For this review, take the finished solid that the model builds, in its own axes (mm). Face numbers are marked on the shaded views. A direction names the side the tool comes from. Give positions to 0.01 mm unless a question says otherwise; leave off trailing zeros. Loops run counter-clockwise (first coordinate to the right, second up) from the corner with the lowest first, then second, coordinate; pieces in that order, holes last.
```python
from build123d import *

# Parameters (mm, degrees)
CROQUIS1_R              = 4
SALIENTE_EXTRUIR1_DEPTH = 3
REDONDEO1_R             = 1
CROQUIS2_W              = 2
CROQUIS2_H              = 10.515557436
CORTAR_EXTRUIR1_DEPTH   = 1
CROQUIS3_R              = 1.75
SALIENTE_EXTRUIR2_DEPTH = 15
CHAFL_N1_SIZE           = 2.47
CHAFL_N1_SIZE2          = 1.729512619


with BuildPart() as part:
    # Croquis1 → Saliente-Extruir1 (new body)
    with BuildSketch(Plane.XY):
        Circle(CROQUIS1_R)
    extrude(amount=SALIENTE_EXTRUIR1_DEPTH)

    # Redondeo1
    redondeo1_edges = [part.edges().sort_by_distance(p)[0] for p in [
        (-4, 0, 0),
        (-4, 0, 3),
    ]]
    fillet(redondeo1_edges, radius=REDONDEO1_R)

    # Croquis2 → Cortar-Extruir1 (cut)
    with BuildSketch(Plane.XY.offset(3)):
        Rectangle(CROQUIS2_W, CROQUIS2_H)
    extrude(amount=-CORTAR_EXTRUIR1_DEPTH, mode=Mode.SUBTRACT)

    # Croquis3 → Saliente-Extruir2 (add)
    with BuildSketch(Plane(origin=(0, 0, 0), x_dir=(-1, 0, 0), z_dir=(0, 0, -1))):
        with Locations(Location((0, 0, 0), (0, 0, 180))):
            Circle(CROQUIS3_R)
    extrude(amount=SALIENTE_EXTRUIR2_DEPTH)

    # Chaflán1
    chafl_n1_edges = [part.edges().sort_by_distance(p)[0] for p in [
        (-1.75, 0, -15),
    ]]
    chafl_n1_side = [part.faces().sort_by_distance(p)[0] for p in [
        (-1.75, 0, -7.5),
    ]]
    chamfer(chafl_n1_edges, length=CHAFL_N1_SIZE, length2=CHAFL_N1_SIZE2, reference=chafl_n1_side[0])


solid = part.part
```
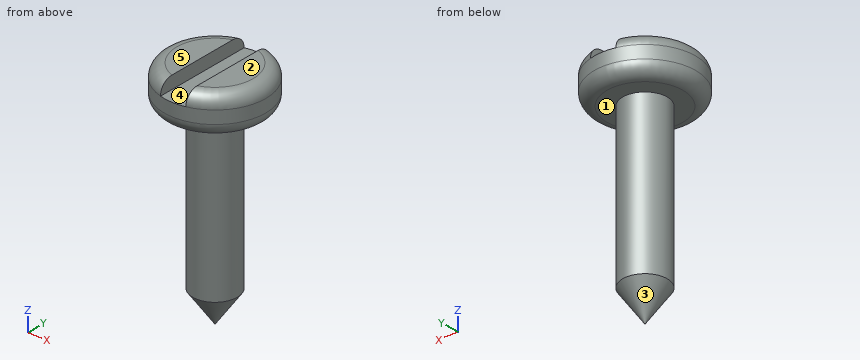
Q1. Mouldability with a two-part tool opening along X and no side actions: class the marked faces 3, 4 and 5 as +X half, -X half, draft (parallel to the pull), parting line (faces both ways), or undercut.
Answers:
face 3: parting line
face 4: undercut
face 5: draft
Q2. Consider section A-A on z = -9.5. Give the boundary of the cut face in (x, y), plus the area to 3 significant figures.
Answers:
outline: circle Ø3.5 at (0, 0)
area: 9.62 mm2
Q3. For pin 1 Ø1 at (y, z) = (-1.5, -7) entering from -X; pin 2 Ø1.5 at (x, y) = (-3, 2.5) entering from -Z; pin 3 Ø1 at (x, z) = (-1, -2) entering from +Y; pin 4 Ø2 at (x, y) = (-0.5, -0.5) entering from +Z, all flat-tipped, find the tip position at first contact; note any pin that passes through.
Answers:
pin 1: stops at x = -1.44
pin 2: stops at z = 0.01
pin 3: stops at y = 1.68
pin 4: stops at z = 3
Q4. Machinability: for the marked faces 1 and 2, which of the approach directions +Z, -Z, +X, -X, +Y, -Y give a long, thin tool a straight path to every point of the face, cutting with its end or side? Answer none if there is none.
Answers:
face 1: -Z
face 2: +Z, +X, -X, +Y, -Y
Q5. For probe 1 along Z at (x, y) = (-1.5, -2.25); probe 2 along Z at (x, y) = (-0.5, 3); probe 3 along Y at (x, z) = (0, -4.75), list the stretches that pass through material, from the lowest coordinate up.
Answers:
probe 1: z = 0 to 3
probe 2: z = 0 to 2
probe 3: y = -1.75 to 1.75
